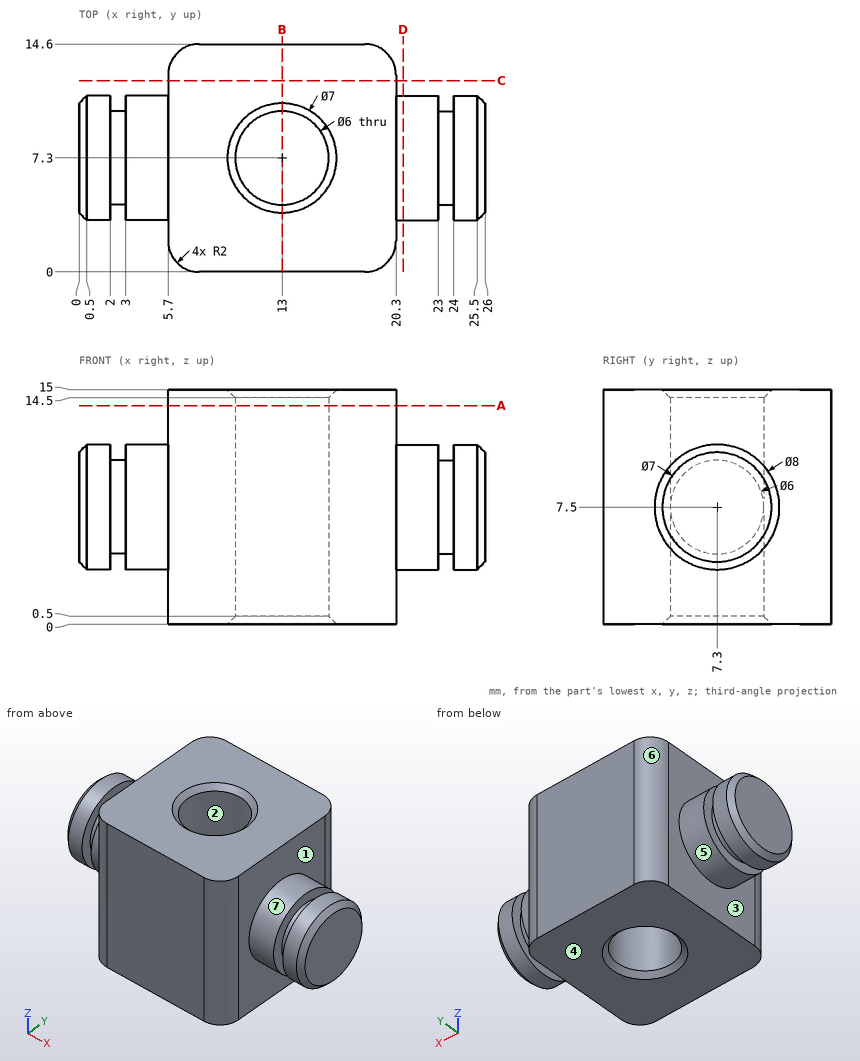
Design review of the part shown in the three views and the two pictorial views. Dimensions are in mm from the part's minimum x, y and z. A direction names the side the tool comes from. Coordinates: 2 decimals unless noted, no trailing zeros. Loops run counter-clockwise (first coordinate to the right, second up) from the corner with the lowest first, then second, coordinate; pieces in that order, holes last.
Q1. Tool access review of the marked faces 5, 6 and 7: name each direction out of +Z, -Z, +X, -X, +Y, -Y from which nothing blocks a thin tool from reaching the whole face with its end or side.
Reported:
face 5: -X
face 6: +Z, -Z, -X, +Y
face 7: +X
Q2. The part is to be moulded in two halves that separate along X. For the marked faces 1, 2, 3 and 4, say which applies: +X half, -X half, draft (parallel to the pull), parting line (faces both ways), or undercut.
Reported:
face 1: +X half
face 2: undercut
face 3: -X half
face 4: draft
Q3. We need section C-C on y = 12.25. State the section outline as (x, z) points.
Reported:
outline: (5.7, 0) - (20.3, 0) - (20.3, 15) - (5.7, 15) - close
Q4. We need section D-D on x = 20.75. State the section outline as (y, z) points, and give its area (3 significant figures).
Reported:
outline: circle Ø8 at (7.3, 7.5)
area: 50.3 mm2
Q5. We need section A-A on z = 14. State the section outline as (x, y) points.
Reported:
outline: (5.7, 2) arc R2 ccw to (7.7, 0) - (18.3, 0) arc R2 ccw to (20.3, 2) - (20.3, 12.6) arc R2 ccw to (18.3, 14.6) - (7.7, 14.6) arc R2 ccw to (5.7, 12.6) - close; hole circle Ø6 at (13, 7.3)
Q6. To check wall thickness, follow line 1 (X direction, y = 10.5, z = 6.75); line 2 (Y direction, x = 13, z = 8.5); line 3 (X direction, y = 10, z = 2.25). State the ranges of each line that lie inside material, in increasing order.
Reported:
line 1: x = 0 to 2, 3 to 23, 24 to 26
line 2: y = 0 to 4.3, 10.3 to 14.6
line 3: x = 5.7 to 11.69, 14.31 to 20.3
Q7. For pin 1 (2 mm diameter, centred on y = 10, z = 12.5, fed in from -X), flat-tipped, find the tip position at first contact; note if it passes through.
Reported:
pin 1: stops at x = 5.7
Q8. We need section B-B on x = 13. State the section outline as (y, z) points, and give its area (4 significant figures).
Reported:
outline: (0, 0) - (3.8, 0) - (4.3, 0.5) - (4.3, 14.5) - (3.8, 15) - (0, 15) - close; (10.3, 0.5) - (10.8, 0) - (14.6, 0) - (14.6, 15) - (10.8, 15) - (10.3, 14.5) - close
area: 128.5 mm2
